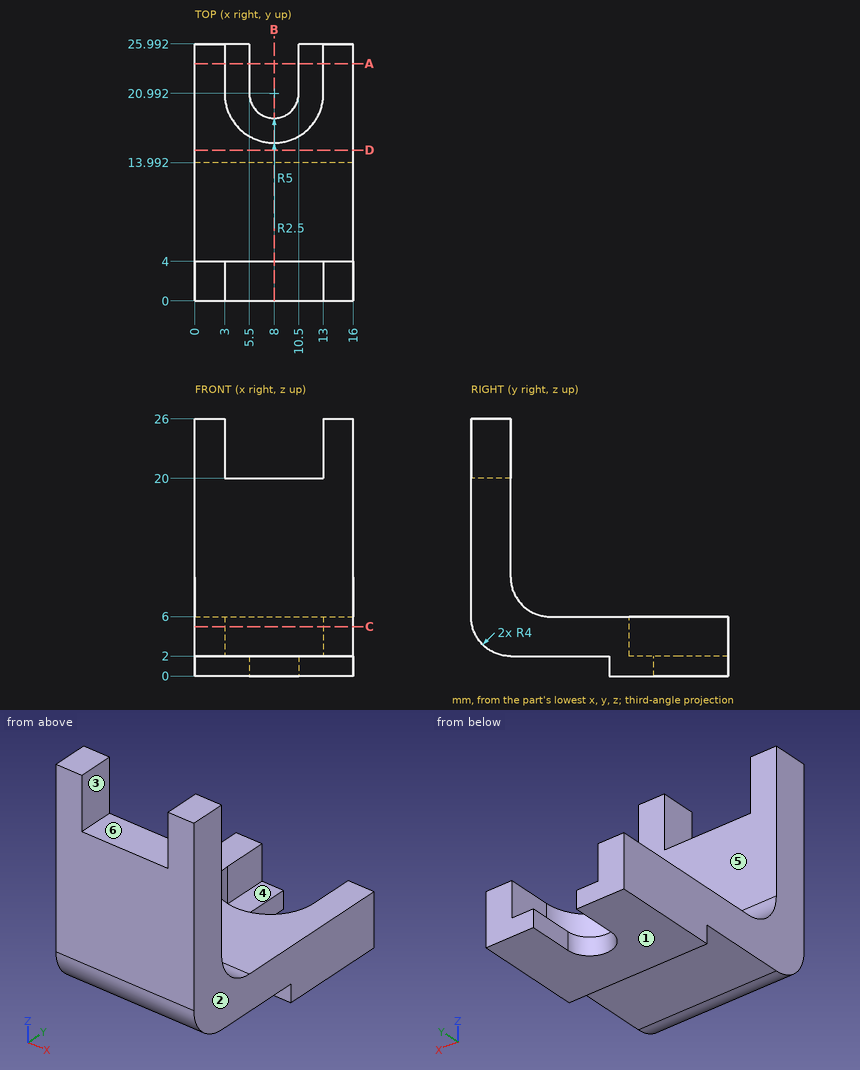
Drawing for the job (mm, zero at the part's lowest x, y, z). A direction names the side the tool comes from. Give positions to 0.01 mm unless a question says otherwise; leave off trailing zeros. Loops run counter-clockwise (first coordinate to the right, second up) from the corner with the lowest first, then second, coordinate; pieces in that order, holes last.
1) Band-saw the part on C-C on z = 5. List the corners of the cut face in (x, y).
Values follow:
outline: (0, 0.13) - (16, 0.13) - (16, 25.99) - (13, 25.99) - (13, 20.99) arc R5 cw to (3, 20.99) - (3, 25.99) - (0, 25.99) - close
2) Probe line 1 along X through (y, z) = (23.5, 3.5); line 2 along Y through (x, z) = (7.25, 14.75); line 3 along Z through (x, y) = (4.5, 9.5). List the from-to ranges inside material, lowest first.
Values follow:
line 1: x = 0 to 3, 13 to 16
line 2: y = 0 to 4
line 3: z = 2 to 6
3) Band-saw the part on B-B on x = 8. List the corners of the cut face in (y, z), then the cut area to 3 significant figures.
Values follow:
outline: (0, 6) arc R4 ccw to (4, 2) - (13.99, 2) - (13.99, 0) - (18.49, 0) - (18.49, 2) - (15.99, 2) - (15.99, 6) - (8, 6) arc R4 cw to (4, 10) - (4, 20) - (0, 20) - close
area: 129 mm2
4) Band-saw the part on D-D on y = 15.25. List the corners of the cut face in (x, z), then the cut area to 3 significant figures.
Values follow:
outline: (0, 0) - (16, 0) - (16, 6) - (0, 6) - close
area: 96.0 mm2
5) Two-plate mould, pull along X, no slides. Class the marked faces 1, 2 and 3: released by +X, released by -X, zero draft, split by the parting line, or undercut.
Values follow:
face 1: zero draft
face 2: released by +X
face 3: undercut
6) Drop flat-ended pins along their axis: P1, Ø8, axis at x = 8, y = 10.5, coming from the -Z side; P2, Ø8, axis at x = 6.5, z = 14, coming from the +Y side; P3, Ø6, axis at x = 13, y = 8.5, coming from the +Z side; P4, Ø1.2, axis at x = 9.5, y = 3, coming from the +Z side. Give the stop position or say it passes through.
Values follow:
P1: stops at z = 0
P2: stops at y = 4
P3: stops at z = 6.88
P4: stops at z = 20
7) Band-saw the part on A-A on y = 24. List the corners of the cut face in (x, z).
Values follow:
outline: (0, 0) - (5.5, 0) - (5.5, 2) - (3, 2) - (3, 6) - (0, 6) - close; (10.5, 0) - (16, 0) - (16, 6) - (13, 6) - (13, 2) - (10.5, 2) - close
8) 3-axis set-ups, long thin cutter, end or side, ignore diameter. For the marked faces 4, 5 and 6: which of +Z, -Z, +X, -X, +Y, -Y reach the whole face in a straight line?
Values follow:
face 4: +Z, +Y
face 5: +Z, +X, -X, +Y
face 6: +Z, +Y, -Y
